The figure shows three views and two pictorial views of one solid part (mm, origin at its lowest corner). Answer the questions. Round coordinates to 2 decimals unless told otherwise and drop trailing zeros. Order: outer loops, then holes, each group sorted by start corner. A loop starts at its lowest first (then second) coordinate and runs counter-clockwise, first axis right, second up. Notation, with made-up numbers: M 68,82.25 L 78,82.25 A21 cw 78,111.25 Z; hole C 36.25,-37 d5. An arc over 180 degrees is marked long. Return JSON: item names as keys, results as strings.
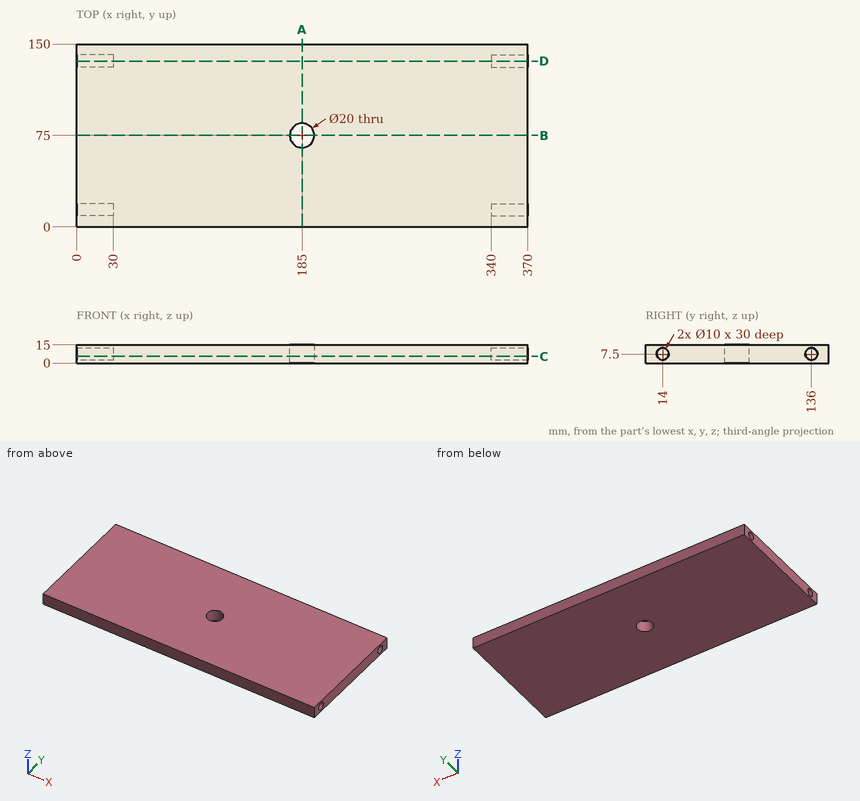
Item 1: Find section D-D (y = 136). Determine the outline of the cut face in (x, z).
Output:
{"outline": "M 0,0 L 370,0 L 370,2.5 L 340,2.5 L 340,12.5 L 370,12.5 L 370,15 L 0,15 L 0,12.5 L 30,12.5 L 30,2.5 L 0,2.5 Z"}
Item 2: Find section C-C (z = 5.5). Determine the outline of the cut face in (x, y).
Output:
{"outline": "M 0,0 L 370,0 L 370,9.42 L 340,9.42 L 340,18.58 L 370,18.58 L 370,131.42 L 340,131.42 L 340,140.58 L 370,140.58 L 370,150 L 0,150 L 0,140.58 L 30,140.58 L 30,131.42 L 0,131.42 L 0,18.58 L 30,18.58 L 30,9.42 L 0,9.42 Z; hole C 185,75 d20"}
Item 3: Consider line 1 along Y through (x, z) = (15.5, 7.5); line 2 along Z through (x, y) = (355.5, 136); line 3 along X through (y, z) = (12.5, 8). Determine where each line is inside the solid, lowest interval first. Write a range as [from, to].
Output:
{"line 1": "y = [0, 9], [19, 131], [141, 150]", "line 2": "z = [0, 2.5], [12.5, 15]", "line 3": "x = [30, 340]"}
Item 4: Each of these flat-tipped pins is pushed along its axis until it touches: pin 1 (3 mm diameter, centred on y = 134, z = 6.5, fed in from +X); pin 2 (8 mm diameter, centred on y = 14, z = 7.5, fed in from -X). Where does it stop, or does it pass through?
Output:
{"pin 1": "stops at x = 340", "pin 2": "stops at x = 30"}
Item 5: Find section B-B (y = 75). Determine the outline of the cut face in (x, z).
Output:
{"outline": "M 0,0 L 175,0 L 175,15 L 0,15 Z; M 195,0 L 370,0 L 370,15 L 195,15 Z"}
Item 6: Find section A-A (x = 185). Determine the outline of the cut face in (y, z).
Output:
{"outline": "M 0,0 L 65,0 L 65,15 L 0,15 Z; M 85,0 L 150,0 L 150,15 L 85,15 Z"}
